Design review of the part built by this model. Coordinates are the model's own, in mm. Face numbers are marked on the shaded views. Coordinates: 2 decimals unless noted, no trailing zeros. Write each loop counter-clockwise with the first axis right and the second up, starting at its lowest first coordinate (ties: lowest second). Pieces come first, ordered by that corner, then holes. Notation, with made-up numbers: (32, -13) - (41, -13) arc R25 ccw to (41, 17) - close; hole circle Ø3 at (78, 49). An arc over 180 degrees is marked (long way). One line per item, written item: value.
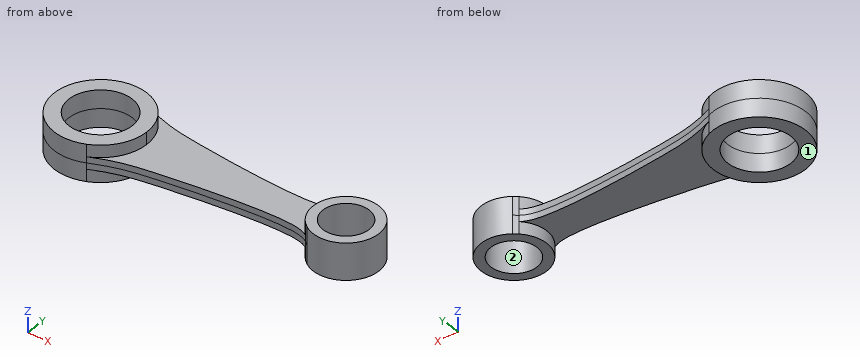
from build123d import *

# Parameters (mm, degrees)
F0_R          = 9.5
F1_DEPTH      = 7.5
F1_DEPTH_BACK = 7.5
F2_DEPTH      = 2.5
F2_DEPTH_BACK = 2.5
F0_R_2        = 13
F3_DEPTH      = 7.5
F3_DEPTH_BACK = 7.5


with BuildPart() as f1:
    # F0 (on Top) → F1 (new body, two sides)
    with BuildSketch(Plane.XY) as f1_sk:
        with BuildLine():
            add(Edge.make_bspline(
                [(43.9010166471, 9.5806238455), (44.5485219286, 10.0415760161), (45.0751125089, 10.5266840027), (45.5859115044, 11)],
                knots=[0.9350422263, 0.9350422263, 0.9350422263, 0.9350422263, 1, 1, 1, 1], degree=3))
            ThreePointArc((43.9010166471, 9.5806238455), (39.9121494256, 0), (43.9010166471, -9.5806238455))
            add(Edge.make_bspline(
                [(43.9010166471, -9.5806238455), (44.5485219286, -10.0415760161), (45.0751125089, -10.5266840027), (45.5859115044, -11)],
                knots=[0.9350422263, 0.9350422263, 0.9350422263, 0.9350422263, 1, 1, 1, 1], degree=3))
            ThreePointArc((45.5859115044, -11), (59.6006786557, -11.9980042494), (66.9121494256, 0))
            ThreePointArc((66.9121494256, 0), (59.6006786557, 11.9980042494), (45.5859115044, 11))
        make_face()
        with Locations((53.4121494256, 0)):
            Circle(F0_R, mode=Mode.SUBTRACT)
    extrude(amount=F1_DEPTH)
    extrude(f1_sk.sketch, amount=-F1_DEPTH_BACK)

    # F0 (on Top) → F2 (join, two sides)
    with BuildSketch(Plane.XY) as f2_sk:
        with BuildLine():
            ThreePointArc((-41.0227190043, 17.4289639487), (-32.7017324231, 10.4226316295), (-29.5878505744, 0))
            ThreePointArc((-29.5878505744, 0), (-32.7017324231, -10.4226316295), (-41.0227190043, -17.4289639487))
            add(Edge.make_bspline(
                [(-41.0227190043, -17.4289639487), (-31.8343407137, -13.4407010268), (-20.2692157487, -11.0133845608), (34.5806966737, -4.8452402532), (42.7048954376, -8.7291177906), (43.9010166471, -9.5806238455)],
                knots=[0, 0, 0, 0, 0.3290608689, 0.8150472654, 0.9350422263, 0.9350422263, 0.9350422263, 0.9350422263], degree=3))
            ThreePointArc((43.9010166471, -9.5806238455), (39.9121494256, 0), (43.9010166471, 9.5806238455))
            add(Edge.make_bspline(
                [(-41.0227190043, 17.4289639487), (-31.8343407137, 13.4407010268), (-20.2692157487, 11.0133845608), (34.5806966737, 4.8452402532), (42.7048954376, 8.7291177906), (43.9010166471, 9.5806238455)],
                knots=[0, 0, 0, 0, 0.3290608689, 0.8150472654, 0.9350422263, 0.9350422263, 0.9350422263, 0.9350422263], degree=3))
        make_face()
    extrude(amount=F2_DEPTH)
    extrude(f2_sk.sketch, amount=-F2_DEPTH_BACK)

    # F0 (on Top) → F3 (join, two sides)
    with BuildSketch(Plane.XY) as f3_sk:
        with BuildLine():
            ThreePointArc((-41.0227190043, -17.4289639487), (-32.7017324231, -10.4226316295), (-29.5878505744, 0))
            ThreePointArc((-29.5878505744, 0), (-32.7017324231, 10.4226316295), (-41.0227190043, 17.4289639487))
            ThreePointArc((-41.0227190043, 17.4289639487), (-67.5878505744, 0), (-41.0227190043, -17.4289639487))
        make_face()
        with Locations((-48.5878505744, 0)):
            Circle(F0_R_2, mode=Mode.SUBTRACT)
    extrude(amount=F3_DEPTH)
    extrude(f3_sk.sketch, amount=-F3_DEPTH_BACK)


solid = f1.part
1. Insertion check: pin 1 Ø3 at (y, z) = (11.5, 5.5) entering from -X; pin 2 Ø2 at (y, z) = (10.5, -4.5) entering from +X; pin 3 Ø1 at (y, z) = (0, -2) entering from -X; pin 4 Ø15 at (x, y) = (53.41, 0) entering from -Z. Each pin has a flat end and moves straight along its axis. Give the tip position at first contact, or say it passes through.
Answer block:
pin 1: stops at x = -64.74
pin 2: stops at x = 63
pin 3: stops at x = -67.59
pin 4: passes through
2. Consider section D-D, the plane x = 58. Write out the cut boundary in (y, z), then the cut area to 3 significant figures.
Answer block:
outline: (-12.7, -7.5) - (-8.32, -7.5) - (-8.32, 7.5) - (-12.7, 7.5) - close; (8.32, -7.5) - (12.7, -7.5) - (12.7, 7.5) - (8.32, 7.5) - close
area: 131 mm^2
3. Wall thickness on line 1 along X through (y, z) = (7.5, 5.75); line 2 along X through (y, z) = (-2, 0.25); line 3 along Y through (x, z) = (-44, 7): over which ranges is each line inside the solid? List them lowest first.
Answer block:
line 1: x = -66.04 to -59.21, -37.97 to -31.13, 42.19 to 47.58, 59.24 to 64.64
line 2: x = -67.48 to -61.43, -35.74 to 44.13, 62.7 to 66.76
line 3: y = -18.44 to -12.16, 12.16 to 18.44
4. Consider section C-C, the plane z = -5.25. Give the number of separate pieces and of enclosed holes in the cut face, then the cut area to 3 significant figures.
Answer block:
separate pieces: 2
enclosed holes: 2
area: 892 mm^2
5. Consider section B-B, the plane x = -49. Write out the cut boundary in (y, z).
Answer block:
outline: (-19, -7.5) - (-12.99, -7.5) - (-12.99, 7.5) - (-19, 7.5) - close; (12.99, -7.5) - (19, -7.5) - (19, 7.5) - (12.99, 7.5) - close
6. Mouldability with a two-part tool opening along X and no side actions: class the marked faces 1 and 2 as released by +X, released by -X, zero draft, split by the parting line, or undercut.
Answer block:
face 1: zero draft
face 2: undercut
7. Consider section A-A, the plane y = 3. Write out the cut boundary in (x, z).
Answer block:
outline: (-67.35, -7.5) - (-61.24, -7.5) - (-61.24, 7.5) - (-67.35, 7.5) - close; (-35.94, -7.5) - (-29.83, -7.5) - (-29.83, -2.5) - (40.25, -2.5) - (40.25, -7.5) - (44.4, -7.5) - (44.4, 7.5) - (40.25, 7.5) - (40.25, 2.5) - (-29.83, 2.5) - (-29.83, 7.5) - (-35.94, 7.5) - close; (62.43, -7.5) - (66.57, -7.5) - (66.57, 7.5) - (62.43, 7.5) - close
